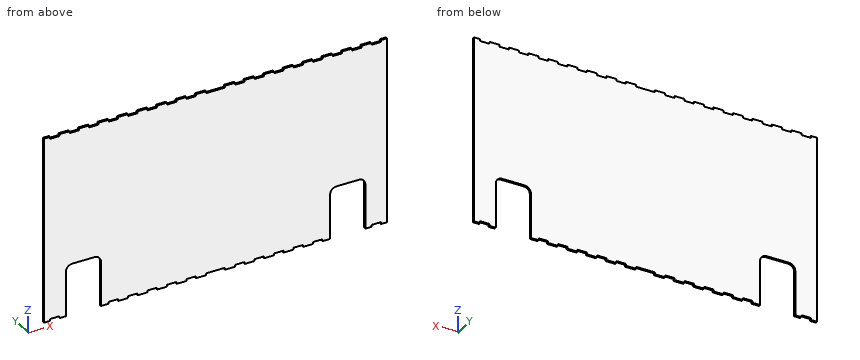
from build123d import *

# Parameters (mm, degrees)
BOSS_EXTRUDE1_DEPTH = 3
FILLET1_R           = 10
SKETCH2_W           = 15
SKETCH2_H           = 3
CUT_EXTRUDE2_DEPTH  = 306.165938466


with BuildPart() as part:
    # Sketch1 → Boss-Extrude1 (new body)
    with BuildSketch(Plane(origin=(0, 0, 0), x_dir=(1, 0, 0), z_dir=(0, 1, 0))):
        Polygon((-234.5, 145), (-268.5, 145), (-268.5, -145), (268.5, -145), (268.5, 145), (234.5, 145), (234.5, 65), (179.5, 65), (179.5, 145), (-179.5, 145), (-179.5, 65), (-234.5, 65), align=None)
    extrude(amount=BOSS_EXTRUDE1_DEPTH)

    # Fillet1
    fillet1_edges = [part.edges().sort_by_distance(p)[0] for p in [
        (-234.5, 1.5, -65),
        (-179.5, 1.5, -65),
        (179.5, 1.5, -65),
        (234.5, 1.5, -65),
    ]]
    fillet(fillet1_edges, radius=FILLET1_R)

    # Sketch2 → Cut-Extrude2 (cut, through all)
    with BuildSketch(Plane(origin=(0, 3, 0), x_dir=(1, 0, 0), z_dir=(0, 1, 0))):
        with Locations((-251.5, 143.5)):
            Rectangle(SKETCH2_W, SKETCH2_H)
        with Locations((-221, 143.5)):
            Rectangle(SKETCH2_W, SKETCH2_H)
        with Locations((-190.5, 143.5)):
            Rectangle(SKETCH2_W, SKETCH2_H)
        with Locations((-160, 143.5)):
            Rectangle(SKETCH2_W, SKETCH2_H)
        with Locations((-129.5, 143.5)):
            Rectangle(SKETCH2_W, SKETCH2_H)
        with Locations((-99, 143.5)):
            Rectangle(SKETCH2_W, SKETCH2_H)
        with Locations((-68.5, 143.5)):
            Rectangle(SKETCH2_W, SKETCH2_H)
        with Locations((-38, 143.5)):
            Rectangle(SKETCH2_W, SKETCH2_H)
        with Locations((-7.5, 143.5)):
            Rectangle(SKETCH2_W, SKETCH2_H)
        with Locations((7.5, 143.5)):
            Rectangle(SKETCH2_W, SKETCH2_H)
        with Locations((38, 143.5)):
            Rectangle(SKETCH2_W, SKETCH2_H)
        with Locations((68.5, 143.5)):
            Rectangle(SKETCH2_W, SKETCH2_H)
        with Locations((99, 143.5)):
            Rectangle(SKETCH2_W, SKETCH2_H)
        with Locations((129.5, 143.5)):
            Rectangle(SKETCH2_W, SKETCH2_H)
        with Locations((160, 143.5)):
            Rectangle(SKETCH2_W, SKETCH2_H)
        with Locations((190.5, 143.5)):
            Rectangle(SKETCH2_W, SKETCH2_H)
        with Locations((221, 143.5)):
            Rectangle(SKETCH2_W, SKETCH2_H)
        with Locations((251.5, 143.5)):
            Rectangle(SKETCH2_W, SKETCH2_H)
        with Locations((-251.5, -143.5)):
            Rectangle(SKETCH2_W, SKETCH2_H)
        with Locations((-221, -143.5)):
            Rectangle(SKETCH2_W, SKETCH2_H)
        with Locations((-190.5, -143.5)):
            Rectangle(SKETCH2_W, SKETCH2_H)
        with Locations((-160, -143.5)):
            Rectangle(SKETCH2_W, SKETCH2_H)
        with Locations((-129.5, -143.5)):
            Rectangle(SKETCH2_W, SKETCH2_H)
        with Locations((-99, -143.5)):
            Rectangle(SKETCH2_W, SKETCH2_H)
        with Locations((-68.5, -143.5)):
            Rectangle(SKETCH2_W, SKETCH2_H)
        with Locations((-38, -143.5)):
            Rectangle(SKETCH2_W, SKETCH2_H)
        with Locations((-7.5, -143.5)):
            Rectangle(SKETCH2_W, SKETCH2_H)
        with Locations((7.5, -143.5)):
            Rectangle(SKETCH2_W, SKETCH2_H)
        with Locations((38, -143.5)):
            Rectangle(SKETCH2_W, SKETCH2_H)
        with Locations((68.5, -143.5)):
            Rectangle(SKETCH2_W, SKETCH2_H)
        with Locations((99, -143.5)):
            Rectangle(SKETCH2_W, SKETCH2_H)
        with Locations((129.5, -143.5)):
            Rectangle(SKETCH2_W, SKETCH2_H)
        with Locations((160, -143.5)):
            Rectangle(SKETCH2_W, SKETCH2_H)
        with Locations((190.5, -143.5)):
            Rectangle(SKETCH2_W, SKETCH2_H)
        with Locations((221, -143.5)):
            Rectangle(SKETCH2_W, SKETCH2_H)
        with Locations((251.5, -143.5)):
            Rectangle(SKETCH2_W, SKETCH2_H)
    extrude(amount=-CUT_EXTRUDE2_DEPTH, mode=Mode.SUBTRACT)


solid = part.part
Model file for the job. Use its own axes, mm. Coordinates: 2 decimals unless noted, no trailing zeros. Write each loop counter-clockwise with the first axis right and the second up, starting at its lowest first coordinate (ties: lowest second). Pieces come first, ordered by that corner, then holes. Notation, with made-up numbers: (62.5, -16) -> (87.5, -16) arc R29 cw to (87.5, 10) -> close; hole circle Ø6 at (38, -35). An arc over 180 degrees is marked (long way). One line per item, written item: value. Start each with the question number.
1) Slice it at B-B on x = 68.5. Write the cut outline in (y, z), then the cut area to 3 significant figures.
2) Flat gauge pin, fed straight in: pin 1 Ø1.5 at (x, y) = (31.5, 1.5) entering from +Z. Where does the tip first touch, or does it go through?
3) Probe probe 1 along X at (y, z) = (2.1, -87); probe 2 along Z at (x, y) = (133.5, 0.6); probe 3 along Z at (x, y) = (209, 2.35). List the from-to ranges inside material, lowest first.
4) Slice it at A-A on z = -88. Write the cut outline in (x, y), then the cut area to 3 significant figures.
Answers follow:
1. outline: (0, -142) -> (3, -142) -> (3, 142) -> (0, 142) -> close
1. area: 852 mm2
2. pin 1: z = 142
3. probe 1: -268.5 to -234.5, -179.5 to 179.5, 234.5 to 268.5
3. probe 2: -142 to 142
3. probe 3: -65 to 145
4. outline: (-268.5, 0) -> (-234.5, 0) -> (-234.5, 3) -> (-268.5, 3) -> close; (-179.5, 0) -> (179.5, 0) -> (179.5, 3) -> (-179.5, 3) -> close; (234.5, 0) -> (268.5, 0) -> (268.5, 3) -> (234.5, 3) -> close
4. area: 1,280 mm2
